The model under review builds one solid part; all positions refer to its coordinate system, in mm. Coordinates: 2 decimals unless noted, no trailing zeros. Order: outer loops, then holes, each group sorted by start corner. A loop starts at its lowest first (then second) coordinate and runs counter-clockwise, first axis right, second up. Notation, with made-up numbers: (33.25, 47.5) -> (71.25, 47.5) arc R36 ccw to (71.25, 82.5) -> close; hole circle Ø10 at (36.5, -9.75). An arc over 180 degrees is marked (long way). Use one line per item in the form item = value. Start each with the question number.
(1) Take a section at D-D (x = 13). State the section outline as (y, z) points, then the cut area to 3 significant figures.
(2) Insertion check: pin 1 Ø1 at (x, z) = (17, -1.5) entering from +Y; pin 2 Ø1 at (x, z) = (-19, -3.5) entering from +Y. Each pin has a flat end and moves straight along its axis. Give the tip position at first contact, or say it passes through.
(3) Wall thickness on line 1 along Y through (x, z) = (0, -2.05); line 2 along X through (y, z) = (58.5, -4.55); line 3 along Y through (x, z) = (-1, -1.1): over which ranges is each line inside the solid? List them lowest first.
(4) Take a section at A-A (x = 0). State the section outline as (y, z) points.
(5) Take a section at B-B (z = -2.15). State the section outline as (x, y) points, then the cut area to 3 significant figures.
(6) Take a section at C-C (y = 61). State the section outline as (x, z) points, then the cut area to 3 significant figures.
```python
from build123d import *

# Parameters (mm, degrees)
BOSS_EXTRUDE1_DEPTH = 5
SKETCH2_R           = 2.5
CUT_EXTRUDE1_DEPTH  = 50


with BuildPart() as part:
    # Sketch1 → Boss-Extrude1 (new body)
    with BuildSketch(Plane.XY):
        with BuildLine():
            ThreePointArc((24.9, 60), (0, 84.9), (-24.9, 60))
            Line((-24.9, 60), (24.9, 60))
        make_face()
        with BuildLine():
            Line((24.9, 60), (-24.9, 60))
            ThreePointArc((-24.9, 60), (0, 35.1), (24.9, 60))
        make_face()
        with BuildLine():
            Line((-24.9, 60), (-24.9, 0))
            Line((-24.9, 0), (24.9, 0))
            Line((24.9, 0), (24.9, 60))
            ThreePointArc((24.9, 60), (0, 35.1), (-24.9, 60))
        make_face()
    extrude(amount=-BOSS_EXTRUDE1_DEPTH)

    # Sketch2 → Cut-Extrude1 (cut)
    with BuildSketch(Plane.XY):
        with Locations((0, 60)):
            Circle(SKETCH2_R)
    extrude(amount=-CUT_EXTRUDE1_DEPTH, mode=Mode.SUBTRACT)


solid = part.part
```
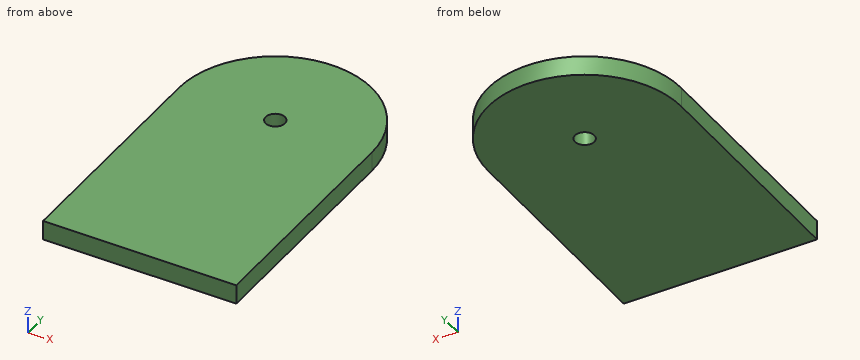
Findings:
q1.outline = (0, -5) -> (81.24, -5) -> (81.24, 0) -> (0, 0) -> close
q1.area = 406 mm²
q2.pin_1 = 78.65
q2.pin_2 = 76.67
q3.line_1 = 0 to 57.5, 62.5 to 84.9
q3.line_2 = -24.9 to -2, 2 to 24.9
q3.line_3 = 0 to 57.71, 62.29 to 84.88
q4.outline = (0, -5) -> (57.5, -5) -> (57.5, 0) -> (0, 0) -> close; (62.5, -5) -> (84.9, -5) -> (84.9, 0) -> (62.5, 0) -> close
q5.outline = (-24.9, 0) -> (24.9, 0) -> (24.9, 60) arc R24.9 ccw to (-24.9, 60) -> close; hole circle Ø5 at (0, 60)
q5.area = 3,940 mm²
q6.outline = (-24.88, -5) -> (-2.29, -5) -> (-2.29, 0) -> (-24.88, 0) -> close; (2.29, -5) -> (24.88, -5) -> (24.88, 0) -> (2.29, 0) -> close
q6.area = 226 mm²
